```python
from build123d import *

# Parameters (mm, degrees)
EXTRUDE_1_DEPTH          = 2
EXTRUDE_1_DEPTH_BACK     = 2
SKETCH_1_W               = 15
SKETCH_1_H               = 2
EXTRUDE_2_DEPTH          = 2
EXTRUDE_2_DEPTH_BACK     = 2
CUT_EXTRUDE_1_DEPTH      = 2
CUT_EXTRUDE_1_DEPTH_BACK = 2
EXTRUDE_3_DEPTH          = 1
EXTRUDE_3_DEPTH_BACK     = 1
FILLET_2_R               = 0.2
FILLET_4_R               = 0.2
FILLET_5_R               = 0.2
FILLET_7_R               = 0.1


with BuildPart() as part:
    # 草图1 → 凸台-拉伸1 (new, two sides: drawn at the far end of the back side and taken through both)
    with BuildSketch(Plane.XY.offset(-EXTRUDE_1_DEPTH_BACK)):
        Rectangle(SKETCH_1_W, SKETCH_1_H)
    extrude(amount=EXTRUDE_1_DEPTH + EXTRUDE_1_DEPTH_BACK)

    # 草图2 → 凸台-拉伸2 (add, two sides: drawn at the far end of the back side and taken through both)
    with BuildSketch(Plane.XY.offset(-EXTRUDE_2_DEPTH_BACK)):
        with BuildLine():
            Line((-1.5, -1), (1.5, -1))
            Line((1.5, -1), (1.5, -1.677124344))
            ThreePointArc((1.5, -1.677124344), (1.780042303, -2.088161527), (1.95, -2.555590279))
            Line((1.95, -2.555590279), (1.95, -3.5))
            Line((1.95, -3.5), (-1.95, -3.5))
            Line((-1.95, -3.5), (-1.95, -2.555590279))
            ThreePointArc((-1.95, -2.555590279), (-1.780042303, -2.088161527), (-1.5, -1.677124344))
            Line((-1.5, -1.677124344), (-1.5, -1))
        make_face()
    extrude(amount=EXTRUDE_2_DEPTH + EXTRUDE_2_DEPTH_BACK)

    # 草图3 → 切除-拉伸1 (cut, two sides: drawn at the far end of the back side and taken through both)
    with BuildSketch(Plane(origin=(0, 0, 0), x_dir=(0, 0, -1), z_dir=(1, 0, 0)).offset(-CUT_EXTRUDE_1_DEPTH_BACK)):
        with BuildLine():
            Line((1.5, -1), (1.5, -1.677124344))
            ThreePointArc((1.5, -1.677124344), (1.780042303, -2.088161527), (1.95, -2.555590279))
            Line((1.95, -2.555590279), (1.95, -3.5))
            Line((1.95, -3.5), (2, -3.5))
            Line((2, -3.5), (2, -1))
            Line((2, -1), (1.5, -1))
        make_face()
        with BuildLine():
            Line((-2, -1), (-1.5, -1))
            Line((-1.5, -1), (-1.5, -1.677124344))
            ThreePointArc((-1.5, -1.677124344), (-1.780042303, -2.088161527), (-1.95, -2.555590279))
            Line((-1.95, -2.555590279), (-1.95, -3.5))
            Line((-1.95, -3.5), (-2, -3.5))
            Line((-2, -3.5), (-2, -1))
        make_face()
    extrude(amount=CUT_EXTRUDE_1_DEPTH + CUT_EXTRUDE_1_DEPTH_BACK, mode=Mode.SUBTRACT)

    # 草图4 → 凸台-拉伸3 (add, two sides: drawn at the far end of the back side and taken through both)
    with BuildSketch(Plane.XY.offset(-EXTRUDE_3_DEPTH_BACK)):
        with BuildLine():
            Line((7.5, 1), (-7.5, 1))
            Line((-7.5, 1), (-2.721884275, 5.009315143))
            ThreePointArc((-2.721884275, 5.009315143), (0, 6), (2.721884275, 5.009315143))
            Line((2.721884275, 5.009315143), (7.5, 1))
        make_face()
    extrude(amount=EXTRUDE_3_DEPTH + EXTRUDE_3_DEPTH_BACK)

    # 圆角2
    fillet_2_edges = [part.edges().sort_by_distance(p)[0] for p in [
        (0, 1, -2),
        (-7.5, 0, -2),
        (0, -1, -2),
        (7.5, 0, -2),
        (-7.5, 0, 2),
        (0, 1, 2),
        (7.5, 0, 2),
        (0, -1, 2),
    ]]
    fillet(fillet_2_edges, radius=FILLET_2_R)

    # 圆角4
    # the kernel refuses this fillet: 0.2 mm, written as the material it takes off along each edge
    with BuildSketch(Plane(origin=(7.3, -0.8, -1.8), x_dir=(0, -1, 0), z_dir=(1, 0, 0))) as fillet_4_piece_1_section:
        Polygon((0, 0), (FILLET_4_R, 0), (FILLET_4_R, FILLET_4_R), (0, FILLET_4_R), align=None)
    fillet_4_piece_1 = extrude(amount=FILLET_4_R, mode=Mode.PRIVATE)
    fillet_4_piece_1 = fillet_4_piece_1 - Plane(origin=(7.3, -0.8, -1.8), x_dir=(0, 0.7071067811865475, 0.7071067811865475), z_dir=(1, 0, 0)) * Sphere(FILLET_4_R, mode=Mode.PRIVATE)
    add(fillet_4_piece_1, mode=Mode.SUBTRACT)
    with BuildSketch(Plane(origin=(-7.3, -0.8, -1.8), x_dir=(-1, 0, 0), z_dir=(0, -1, 0))) as fillet_4_piece_2_section:
        Polygon((0, 0), (FILLET_4_R, 0), (FILLET_4_R, FILLET_4_R), (0, FILLET_4_R), align=None)
    fillet_4_piece_2 = extrude(amount=FILLET_4_R, mode=Mode.PRIVATE)
    fillet_4_piece_2 = fillet_4_piece_2 - Plane(origin=(-7.3, -0.8, -1.8), x_dir=(0.7071067811865475, 0, 0.7071067811865475), z_dir=(0, -1, 0)) * Sphere(FILLET_4_R, mode=Mode.PRIVATE)
    add(fillet_4_piece_2, mode=Mode.SUBTRACT)
    with BuildSketch(Plane(origin=(7.3, -0.8, 1.8), x_dir=(0, -1, 0), z_dir=(1, 0, 0))) as fillet_4_piece_3_section:
        Polygon((0, 0), (FILLET_4_R, 0), (FILLET_4_R, -FILLET_4_R), (0, -FILLET_4_R), align=None)
    fillet_4_piece_3 = extrude(amount=FILLET_4_R, mode=Mode.PRIVATE)
    fillet_4_piece_3 = fillet_4_piece_3 - Plane(origin=(7.3, -0.8, 1.8), x_dir=(0, 0.7071067811865475, -0.7071067811865475), z_dir=(1, 0, 0)) * Sphere(FILLET_4_R, mode=Mode.PRIVATE)
    add(fillet_4_piece_3, mode=Mode.SUBTRACT)
    with BuildSketch(Plane(origin=(-7.3, -0.8, 1.8), x_dir=(-1, 0, 0), z_dir=(0, -1, 0))) as fillet_4_piece_4_section:
        Polygon((0, 0), (FILLET_4_R, 0), (FILLET_4_R, -FILLET_4_R), (0, -FILLET_4_R), align=None)
    fillet_4_piece_4 = extrude(amount=FILLET_4_R, mode=Mode.PRIVATE)
    fillet_4_piece_4 = fillet_4_piece_4 - Plane(origin=(-7.3, -0.8, 1.8), x_dir=(0.7071067811865475, 0, -0.7071067811865475), z_dir=(0, -1, 0)) * Sphere(FILLET_4_R, mode=Mode.PRIVATE)
    add(fillet_4_piece_4, mode=Mode.SUBTRACT)
    with BuildSketch(Plane(origin=(-7.5, -1, 1.8), x_dir=(1, 0, 0), z_dir=(0, 0, -1)), Plane(origin=(7.5, -1, 1.8), x_dir=(0, 1, 0), z_dir=(0, 0, -1))) as fillet_4_piece_5:
        with BuildLine():
            CenterArc((FILLET_4_R, -FILLET_4_R), FILLET_4_R, 90, 90)
            Line((0, -FILLET_4_R), (0, 0))
            Line((0, 0), (FILLET_4_R, 0))
        make_face()
    extrude(amount=3.6, mode=Mode.SUBTRACT)

    # 圆角5
    fillet_5_edges = [part.edges().sort_by_distance(p)[0] for p in [
        (5.110942137, 3.004657571, -1),
        (0, 6, -1),
        (5.110942137, 3.004657571, 1),
        (0, 6, 1),
        (-5.110942137, 3.004657571, -1),
        (-5.110942137, 3.004657571, 1),
    ]]
    fillet(fillet_5_edges, radius=FILLET_5_R)

    # 圆角7
    fillet_7_edges = [part.edges().sort_by_distance(p)[0] for p in [
        (0, -3.5, 1.95),
        (1.95, -3.5, 0),
        (-1.95, -3.5, 0),
        (0, -3.5, -1.95),
    ]]
    fillet(fillet_7_edges, radius=FILLET_7_R)


solid = part.part
```
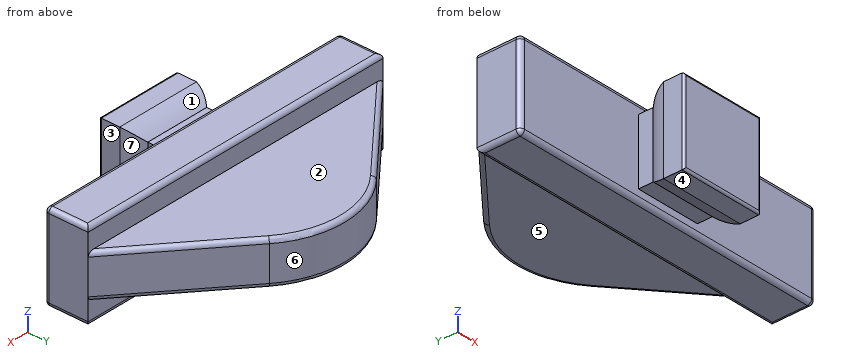
Part model, mm, in its own coordinate system. Face numbers are marked on the shaded views. A direction names the side the tool comes from. Coordinates: 2 decimals unless noted, no trailing zeros. Loops run counter-clockwise (first coordinate to the right, second up) from the corner with the lowest first, then second, coordinate; pieces in that order, holes last. Notation, with made-up numbers: (40.25, 64) - (77.25, 64) arc R15 cw to (77.25, 78) - close; hole circle Ø1 at (18, 7). An arc over 180 degrees is marked (long way). Write item = value, one per line. Start each with the question number.
Item 1: 3-axis set-ups, long thin cutter, end or side, ignore diameter. For the marked faces 1, 2, 3 and 4: which of +Z, -Z, +X, -X, +Y, -Y reach the whole face in a straight line?
Item 2: Flat gauge pins, fed straight in: pin 1 Ø0.5 at (x, z) = (1, 1.5) entering from +Y; pin 2 Ø1.5 at (x, z) = (0.5, -1.5) entering from +Y (3 decimals); pin 3 Ø0.9 at (y, z) = (-3, -0.5) entering from -X. Where does each tip first touch, or does it go through?
Item 3: Wall check: L1, parallel to Y at x = 0.5, z = 1.6; L2, parallel to Z at x = 3.5, y = 2.75. Give the ranges that are in metal, low to high. Write a range as from..to.
Item 4: Cut at A-A, the plane z = -0.25. Give the cut face in (x, y), and give its area (3 significant figures).
Item 5: Mould opens along Y. For the marked faces 5, 6 and 7 say: released by +Y, released by -Y, zero draft, split by the parting line, or undercut.
The answers:
q1.face_1 = +Z, +X, -X
q1.face_2 = +Z, +X, -X, +Y
q1.face_3 = +Z, -Z, +X, -Y
q1.face_4 = -Z, +X, -X, -Y
q2.pin_1 = 1
q2.pin_2 = 5.995
q2.pin_3 = -1.95
q3.L1 = -3.5..-1.8, -1..1
q3.L2 = -1..1
q4.outline = (-7.5, -0.8) arc R0.2 ccw to (-7.3, -1) - (-1.5, -1) - (-1.5, -1.68) arc R2 ccw to (-1.95, -2.56) - (-1.95, -3.4) arc R0.1 ccw to (-1.85, -3.5) - (1.85, -3.5) arc R0.1 ccw to (1.95, -3.4) - (1.95, -2.56) arc R2 ccw to (1.5, -1.68) - (1.5, -1) - (7.3, -1) arc R0.2 ccw to (7.5, -0.8) - (7.5, 1) - (2.72, 5.01) arc R4.23 ccw to (-2.72, 5.01) - (-7.5, 1) - close
q4.area = 83.5 mm2
q5.face_5 = zero draft
q5.face_6 = released by +Y
q5.face_7 = undercut
